Check sheet for the modelled part. Datum: model origin and axes. Units: mm. A direction names the side the tool comes from. Give positions to 0.01 mm unless a question says otherwise; leave off trailing zeros. Write each loop counter-clockwise with the first axis right and the second up, starting at its lowest first coordinate (ties: lowest second). Pieces come first, ordered by that corner, then holes. Notation, with made-up numbers: (78, 31.25) -> (114, 31.25) arc R25 cw to (114, 62.25) -> close; hole circle Ø4 at (82.5, 20.5). An arc over 180 degrees is marked (long way). Answer as a JSON object with one key per item and string values.
Solid Edge part; units mm, degrees
sketch "Sketch1" plane through (0, 0, 0) normal (0, 0, 1) x (1, 0, 0)
  circle A0 centre (32.5, 35) radius 1.5
  line L0 (37.5, 40) -> (-37.5, 40)
  line L1 (-37.5, 40) -> (-37.5, -40)
  line L2 (-37.5, -40) -> (37.5, -40)
  line L3 (37.5, -40) -> (37.5, 40)
  circle A1 centre (-32.5, -35) radius 1.5
  circle A2 centre (-32.5, 35) radius 1.5
  circle A3 centre (32.5, -35) radius 1.5
extrude "Protrusion1" add sketch "Sketch1" along normal blind 1.6
sketch "Sketch2" plane through (0, 0, 1.6) normal (0, 0, 1) x (1, 0, 0)
  line L0 (0.2, -24.5) -> (0.2, -29.5)
  line L1 (0.2, -29.5) -> (-19.3, -29.5)
  line L2 (-19.3, -29.5) -> (-19.3, -24.5)
  line L3 (-19.3, -24.5) -> (0.2, -24.5)
  line L4 (0.2, -16.5) -> (0.2, -21.5)
  line L5 (0.2, -21.5) -> (-19.3, -21.5)
  line L6 (-19.3, -21.5) -> (-19.3, -16.5)
  line L7 (-19.3, -16.5) -> (0.2, -16.5)
  line L8 (0.2, -8.5) -> (0.2, -13.5)
  line L9 (0.2, -13.5) -> (-19.3, -13.5)
  line L10 (-19.3, -13.5) -> (-19.3, -8.5)
  line L11 (-19.3, -8.5) -> (0.2, -8.5)
  line L12 (9, -8) -> (4, -8)
  line L13 (4, -8) -> (4, -30)
  line L14 (4, -30) -> (9, -30)
  line L15 (9, -30) -> (9, -8)
  line L16 (18, -8) -> (13, -8)
  line L17 (13, -8) -> (13, -30)
  line L18 (13, -30) -> (18, -30)
  line L19 (18, -30) -> (18, -8)
  line L20 (27, -8) -> (22, -8)
  line L21 (22, -8) -> (22, -30)
  line L22 (22, -30) -> (27, -30)
  line L23 (27, -30) -> (27, -8)
  line L24 (31, -8) -> (31, -30)
  line L25 (31, -30) -> (36, -30)
  line L26 (36, -30) -> (36, -8)
  line L27 (36, -8) -> (31, -8)
extrude "ExtrudedProtrusion_2" add sketch "Sketch2" along normal blind 19
sketch "Sketch3" plane through (0, 0, 1.6) normal (0, 0, 1) x (1, 0, 0)
  line L0 (-36.5, 5.25) -> (-36.5, -3.75)
  line L1 (-36.5, -3.75) -> (-29, -3.75)
  line L2 (-29, -3.75) -> (-29, 5.25)
  line L3 (-29, 5.25) -> (-36.5, 5.25)
  line L4 (11, 25) -> (-7, 25)
  line L5 (-7, 25) -> (-7, -1)
  line L6 (-7, -1) -> (11, -1)
  line L7 (11, -1) -> (11, 25)
extrude "ExtrudedProtrusion_3" add sketch "Sketch3" along normal blind 3
sketch "Sketch4" plane through (0, 0, 1.6) normal (0, 0, 1) x (1, 0, 0)
  line L0 (-29.5, -8.5) -> (-47.5, -8.5)
  line L1 (-47.5, -8.5) -> (-47.5, -22.5)
  line L2 (-47.5, -22.5) -> (-29.5, -22.5)
  line L3 (-29.5, -22.5) -> (-29.5, -8.5)
  line L4 (-47.5, 10) -> (-29.5, 10)
  line L5 (-29.5, 10) -> (-29.5, 27)
  line L6 (-29.5, 27) -> (-47.5, 27)
  line L7 (-47.5, 27) -> (-47.5, 10)
  line L8 (47.5, 15.5) -> (29.5, 15.5)
  line L9 (29.5, 15.5) -> (29.5, 1.5)
  line L10 (29.5, 1.5) -> (47.5, 1.5)
  line L11 (47.5, 1.5) -> (47.5, 15.5)
extrude "ExtrudedProtrusion_4" add sketch "Sketch4" along normal blind 5
sketch "Sketch5" plane through (0, 0, 1.6) normal (0, 0, 1) x (1, 0, 0)
  line L0 (-18.2995, 5.8505) -> (-24.2995, 5.8505)
  line L1 (-24.2995, 5.8505) -> (-24.2995, 9.8505)
  line L2 (-24.2995, 9.8505) -> (-18.2995, 9.8505)
  line L3 (-18.2995, 9.8505) -> (-18.2995, 5.8505)
  line L4 (13.1657, -4.9907) -> (13.1657, -0.9907)
  line L5 (13.1657, -0.9907) -> (19.1657, -0.9907)
  line L6 (19.1657, -0.9907) -> (19.1657, -4.9907)
  line L7 (19.1657, -4.9907) -> (13.1657, -4.9907)
extrude "ExtrudedProtrusion_5" add sketch "Sketch5" along normal blind 1.5
sketch "Sketch6" plane through (0, 0, 0) normal (0, 0, -1) x (-1, 0, 0)
  line L0 (-36, -8.5) -> (-36, -30)
  line L1 (-36, -30) -> (19.3, -30)
  line L2 (19.3, -30) -> (19.3, -8.5)
  line L3 (19.3, -8.5) -> (-36, -8.5)
extrude "ExtrudedProtrusion_6" add sketch "Sketch6" along normal blind 1
properties material "Polycarbonate"
1. Sectioned sample at D-D, the plane y = 20. Enter the section's corners in (x, z), plus the area to 3 significant figures.
Determined:
{"outline": "(-47.5, 1.6) -> (-37.5, 1.6) -> (-37.5, 0) -> (37.5, 0) -> (37.5, 1.6) -> (11, 1.6) -> (11, 4.6) -> (-7, 4.6) -> (-7, 1.6) -> (-29.5, 1.6) -> (-29.5, 6.6) -> (-47.5, 6.6) -> close", "area": "264 mm^2"}
2. Access from +Z, -Z, +X, -X, +Y, -Y to the whole of each face (thin tool, end or side, straight path). Record for faces 1 (the face through (11, 12, 3)), 2 (the face through (24, -30, 11)), 3 (the face through (-29.5, -16, 4)).
Determined:
{"face 1": "+Z, +Y, -Y", "face 2": "+Z, +X, -X, -Y", "face 3": "+Z, -Y"}
3. Scan lines: L1, parallel to X at y = -22.5, z = 15.75; L2, parallel to Y at x = -4, z = 7.75; L3, parallel to Y at x = -32.5, z = 1.2. Record each from-to range of solid material in increasing order. Write a range as [from, to].
Determined:
{"L1": "[4, 9], [13, 18], [22, 27], [31, 36]", "L2": "[-29.5, -24.5], [-21.5, -16.5], [-13.5, -8.5]", "L3": "[-40, -36.5], [-33.5, 33.5], [36.5, 40]"}
4. Sectioned sample at C-C, the plane z = 18. Enter the section's corners in (x, y), plus the area to 4 significant figures.
Determined:
{"outline": "(-19.3, -29.5) -> (0.2, -29.5) -> (0.2, -24.5) -> (-19.3, -24.5) -> close; (-19.3, -21.5) -> (0.2, -21.5) -> (0.2, -16.5) -> (-19.3, -16.5) -> close; (-19.3, -13.5) -> (0.2, -13.5) -> (0.2, -8.5) -> (-19.3, -8.5) -> close; (4, -30) -> (9, -30) -> (9, -8) -> (4, -8) -> close; (13, -30) -> (18, -30) -> (18, -8) -> (13, -8) -> close; (22, -30) -> (27, -30) -> (27, -8) -> (22, -8) -> close; (31, -30) -> (36, -30) -> (36, -8) -> (31, -8) -> close", "area": "732.5 mm^2"}
5. Sectioned sample at A-A, the plane x = -32.5. Enter the section's corners in (y, z), plus the area to 3 significant figures.
Determined:
{"outline": "(-40, 0) -> (-36.5, 0) -> (-36.5, 1.6) -> (-40, 1.6) -> close; (-33.5, 0) -> (33.5, 0) -> (33.5, 1.6) -> (27, 1.6) -> (27, 6.6) -> (10, 6.6) -> (10, 1.6) -> (5.25, 1.6) -> (5.25, 4.6) -> (-3.75, 4.6) -> (-3.75, 1.6) -> (-8.5, 1.6) -> (-8.5, 6.6) -> (-22.5, 6.6) -> (-22.5, 1.6) -> (-33.5, 1.6) -> close; (36.5, 0) -> (40, 0) -> (40, 1.6) -> (36.5, 1.6) -> close", "area": "300 mm^2"}
6. Go/stop test with flat-tipped pins: P1, Ø1.5, axis at x = 28, z = 16.5, coming from the +Y side; P2, Ø1.8, axis at y = -6.5, z = 0.5, coming from the -X side; P3, Ø4, axis at x = -12.5, z = 15.5, coming from the +Y side; P4, Ø8, axis at x = 45, y = 7, coming from the -Z side. Record where each tip stops, or that it passes through.
Determined:
{"P1": "through", "P2": "x = -37.5", "P3": "y = -8.5", "P4": "z = 1.6"}
7. Sectioned sample at B-B, the plane y = 35. Enter the section's corners in (x, z), plus the area to 3 significant figures.
Determined:
{"outline": "(-37.5, 0) -> (-34, 0) -> (-34, 1.6) -> (-37.5, 1.6) -> close; (-31, 0) -> (31, 0) -> (31, 1.6) -> (-31, 1.6) -> close; (34, 0) -> (37.5, 0) -> (37.5, 1.6) -> (34, 1.6) -> close", "area": "110 mm^2"}
8. Mould release check, pull along Y, two halves, no side actions. Record for faces 4 (the face through (33, -30, 11)), 5 (the face through (-33.7, -34.1, 0.8)), 6 (the face through (9, -19, 11)): released by +Y, released by -Y, zero draft, split by the parting line, or undercut.
Determined:
{"face 4": "released by -Y", "face 5": "undercut", "face 6": "zero draft"}
